from build123d import *

# Parameters (mm, degrees)
SKETCH3_R           = 12.5
BOSS_EXTRUDE1_DEPTH = 74.8
SKETCH4_R           = 5
BOSS_EXTRUDE2_DEPTH = 0.5
SKETCH5_R           = 2
BOSS_EXTRUDE3_DEPTH = 11
SKETCH6_R           = 1.5
CUT_EXTRUDE1_DEPTH  = 4


with BuildPart() as part:
    # Sketch3 → Boss-Extrude1 (new body)
    with BuildSketch(Plane.XY):
        Circle(SKETCH3_R)
    extrude(amount=BOSS_EXTRUDE1_DEPTH)

    # Sketch4 → Boss-Extrude2 (add)
    with BuildSketch(Plane.XY.offset(74.8)):
        Circle(SKETCH4_R)
    extrude(amount=BOSS_EXTRUDE2_DEPTH)

    # Sketch5 → Boss-Extrude3 (add)
    with BuildSketch(Plane.XY.offset(75.3)):
        Circle(SKETCH5_R)
    extrude(amount=BOSS_EXTRUDE3_DEPTH)

    # Sketch6 → Cut-Extrude1 (cut)
    with BuildSketch(Plane.XY.offset(74.8)):
        with Locations((-8.5, 0)):
            Circle(SKETCH6_R)
        with Locations((8.5, 0)):
            Circle(SKETCH6_R)
    extrude(amount=-CUT_EXTRUDE1_DEPTH, mode=Mode.SUBTRACT)


solid = part.part
Here's how the part is built. I have some questions about the finished solid (model axes, mm). A direction names the side the tool comes from. Give positions to 0.01 mm unless a question says otherwise; leave off trailing zeros. Order: outer loops, then holes, each group sorted by start corner. A loop starts at its lowest first (then second) coordinate and runs counter-clockwise, first axis right, second up. Notation, with made-up numbers: (49, 4) -> (63, 4) arc R21 cw to (63, 19) -> close; hole circle Ø5 at (-17, 50.5). An arc over 180 degrees is marked (long way). Use a Markdown table: item, result. Add a question column.
Item 1: Imagine slicing it at D-D on z = 64. Please give me the cut outline in (x, y).
Item 2: For faces 1 (the face through (11.923, 3.755, 36.876)), 2 (the face through (7.3, -0.9, 72.8)), which set-ups out of +Z, -Z, +X, -X, +Y, -Y let a thin tool reach every point of the face, with its end or its side?
Item 3: I need wall thicknesses on line 1 (Z direction, x = -9, y = 4); line 2 (Y direction, x = -8.5, z = 73.7); line 3 (Z direction, x = 3.5, y = -1.5). Which ranges of each line are inside material? Lowest first, please.
Item 4: If we mould it in two halves opening along X, with no side actions, what happens to faces 3 (the face through (0, -2, 81)), 4 (the face through (-0.1, -2.2, 75.3)), 5 (the face through (8, 0, 70.8))? For each: pulls with the +X half, pulls with the -X half, needs draft (parallel to the pull), parting line crosses it, or undercut.
Item 5: Imagine slicing it at A-A on x = 0. Please give me the cut outline in (y, z), plus the area to 3 significant figures.
Item 6: Imagine slicing it at B-B on z = 74. Please give me the cut outline in (x, y).
Item 7: Will these pins go through, and if not, where does the flat tip stop? pin 1 (1.5 mm diameter, centred on x = -9, y = 0.5, fed in from +Z); pin 2 (3.5 mm diameter, centred on x = 8.5, y = -0.5, fed in from +Z); pin 3 (10 mm diameter, centred on x = 0.5, z = 32, fed in from -Y); pin 4 (1 mm diameter, centred on x = -4, y = 3.5, fed in from +Z).
Item 8: Imagine slicing it at C-C on y = 0. Please give me the cut outline in (x, z).
Data:
| question | item | result |
|---|---|---|
| 1 | outline | circle Ø25 at (0, 0) |
| 2 | face 1 | +Z, -Z |
| 2 | face 2 | +Z |
| 3 | line 1 | z = 0 to 74.8 |
| 3 | line 2 | y = -9.17 to -1.5, 1.5 to 9.17 |
| 3 | line 3 | z = 0 to 75.3 |
| 4 | face 3 | parting line crosses it |
| 4 | face 4 | needs draft |
| 4 | face 5 | undercut |
| 5 | outline | (-12.5, 0) -> (12.5, 0) -> (12.5, 74.8) -> (5, 74.8) -> (5, 75.3) -> (2, 75.3) -> (2, 86.3) -> (-2, 86.3) -> (-2, 75.3) -> (-5, 75.3) -> (-5, 74.8) -> (-12.5, 74.8) -> close |
| 5 | area | 1,920 mm² |
| 6 | outline | circle Ø25 at (0, 0); hole circle Ø3 at (-8.5, 0); hole circle Ø3 at (8.5, 0) |
| 7 | pin 1 | stops at z = 70.8 |
| 7 | pin 2 | stops at z = 74.8 |
| 7 | pin 3 | stops at y = -12.5 |
| 7 | pin 4 | stops at z = 75.3 |
| 8 | outline | (-12.5, 0) -> (12.5, 0) -> (12.5, 74.8) -> (10, 74.8) -> (10, 70.8) -> (7, 70.8) -> (7, 74.8) -> (5, 74.8) -> (5, 75.3) -> (2, 75.3) -> (2, 86.3) -> (-2, 86.3) -> (-2, 75.3) -> (-5, 75.3) -> (-5, 74.8) -> (-7, 74.8) -> (-7, 70.8) -> (-10, 70.8) -> (-10, 74.8) -> (-12.5, 74.8) -> close |
